Study the drawing (mm; zero at the part's minimum x, y, z) and answer. Coordinates: 2 decimals unless noted, no trailing zeros. Loops run counter-clockwise (first coordinate to the right, second up) from the corner with the lowest first, then second, coordinate; pieces in that order, holes last. Notation, with made-up numbers: (59.5, -26) -> (108.5, -26) arc R27 cw to (108.5, -6) -> close; hole circle Ø4 at (-22.5, 27). An arc over 180 degrees is marked (long way). Answer as a JSON object with one key per item and string values. Group by question number.
Q1. Each of these flat-tipped pins is pushed along its axis until it touches: P1, Ø1.5, axis at y = 26.5, z = 1, coming from the -X side; P2, Ø1.5, axis at y = 27, z = 1.5, coming from the +X side. Where does it stop, or does it pass through?
Q2. Straight lines are drawn through the part: line 1 along X through (y, z) = (73.5, 2.45); line 2 along Y through (x, z) = (73, 0.3); line 3 along X through (y, z) = (53, 1.5). For each, find the intervals that lie inside material, in ascending order. Write a range as [from, to].
Q3. The part is cut by section B-B on z = 1.6. Write down the section's boundary in (x, y), and give its area (3 significant figures).
Q4. The part is cut by section C-C on x = 67.5. Write down the section's boundary in (y, z).
Q5. The part is cut by section A-A on y = 47. Write down the section's boundary in (x, z).
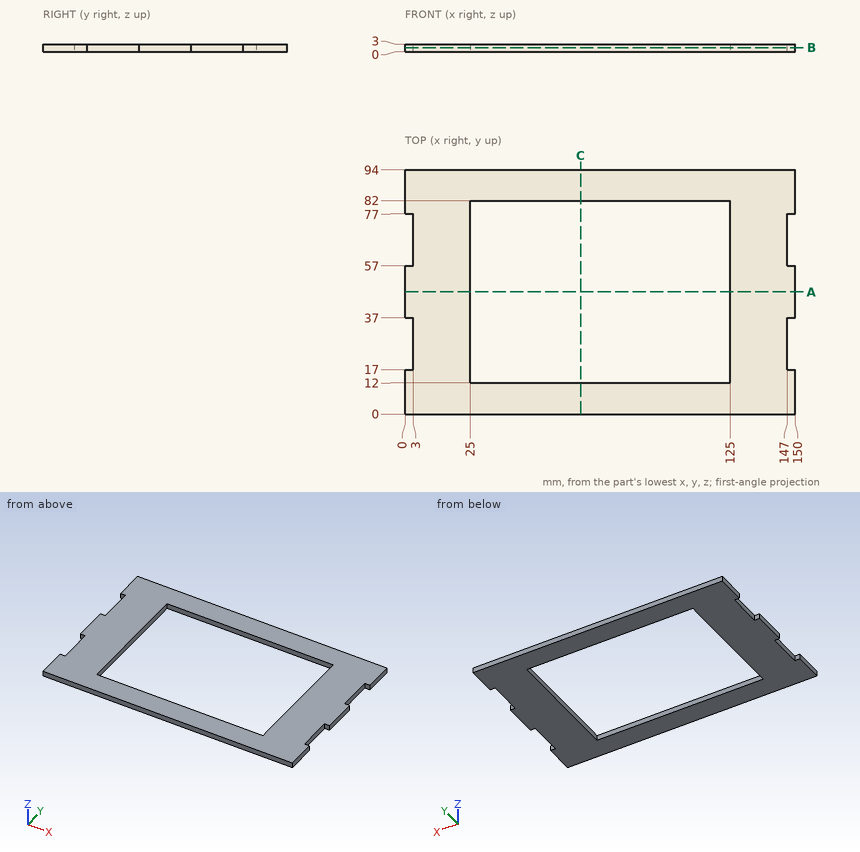
Final values:
{
 "1": {"P1": "stops at x = 3", "P2": "stops at x = 147"},
 "2": {"line 1": "x = [3, 25], [125, 147]", "line 2": "y = [0, 12], [82, 94]", "line 3": "x = [0, 25], [125, 150]"},
 "3": {"outline": "(0, 0) -> (150, 0) -> (150, 17) -> (147, 17) -> (147, 37) -> (150, 37) -> (150, 57) -> (147, 57) -> (147, 77) -> (150, 77) -> (150, 94) -> (0, 94) -> (0, 77) -> (3, 77) -> (3, 57) -> (0, 57) -> (0, 37) -> (3, 37) -> (3, 17) -> (0, 17) -> close; hole (25, 12) -> (125, 12) -> (125, 82) -> (25, 82) -> close", "area": "6,860 mm2"},
 "4": {"outline": "(0, 0) -> (12, 0) -> (12, 3) -> (0, 3) -> close; (82, 0) -> (94, 0) -> (94, 3) -> (82, 3) -> close"},
 "5": {"outline": "(0, 0) -> (25, 0) -> (25, 3) -> (0, 3) -> close; (125, 0) -> (150, 0) -> (150, 3) -> (125, 3) -> close"}
}
